Could you check a few things on this model? Use its own coordinates, in mm. Coordinates: 2 decimals unless noted, no trailing zeros. Loops run counter-clockwise (first coordinate to the right, second up) from the corner with the lowest first, then second, coordinate; pieces in that order, holes last. Notation, with made-up numbers: (10, 37.5) - (44, 37.5) arc R21 ccw to (44, 64.5) - close; hole circle Ø6 at (40.25, 61). An arc over 180 degrees is marked (long way). Use CSV: the item, a comma, the result in double quotes.
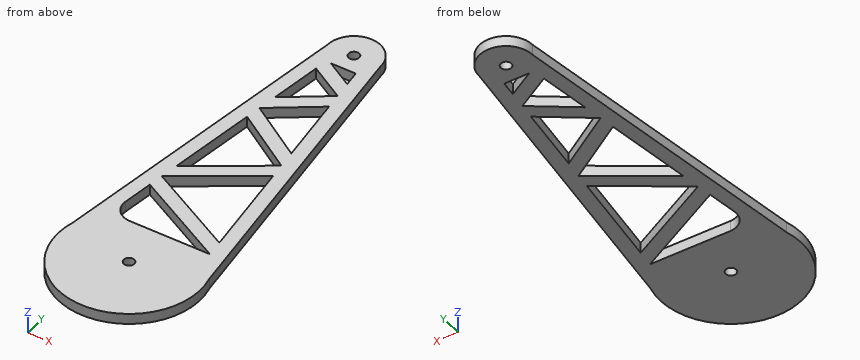
from build123d import *

# Parameters (mm, degrees)
SKETCH1_R           = 1.5
BOSS_EXTRUDE1_DEPTH = 3
FILLET1_R           = 5


with BuildPart() as part:
    # Sketch1 → Boss-Extrude1 (new body)
    with BuildSketch(Plane.XY):
        with BuildLine():
            Line((-19.319264806, 5.173587474), (-7.5, 95))
            ThreePointArc((-7.5, 95), (0, 102.5), (7.5, 95))
            Line((7.5, 95), (19.319264806, 5.173587474))
            ThreePointArc((19.319264806, 5.173587474), (0, -20), (-19.319264806, 5.173587474))
        make_face()
        with Locations((0, 95)):
            Circle(SKETCH1_R, mode=Mode.SUBTRACT)
        Circle(SKETCH1_R, mode=Mode.SUBTRACT)
        Polygon((-14.254996232, 13), (14.254996232, 13), (-12.38556129, 27.207705563), align=None, mode=Mode.SUBTRACT)
        Polygon((-2.898329399, 89.534418399), (4.184678022, 89.534418399), (4.774242146, 85.053731057), align=None, mode=Mode.SUBTRACT)
        Polygon((-11.828187859, 31.443743635), (13.613494732, 17.875411404), (9.904156147, 46.066384645), align=None, mode=Mode.SUBTRACT)
        Polygon((-11.132206149, 36.73320463), (-7.866560771, 61.552109505), (9.321386275, 50.495435676), align=None, mode=Mode.SUBTRACT)
        Polygon((-7.289587852, 65.937103693), (8.637709175, 55.691381633), (6.027006268, 75.532723726), align=None, mode=Mode.SUBTRACT)
        Polygon((-6.572917095, 71.383801447), (5.434465341, 80.036034774), (-4.658887227, 85.930428438), align=None, mode=Mode.SUBTRACT)
    extrude(amount=BOSS_EXTRUDE1_DEPTH)

    # Fillet1
    fillet1_edges = [part.edges().sort_by_distance(p)[0] for p in [
        (-14.254996232, 13, 1.5),
    ]]
    fillet(fillet1_edges, radius=FILLET1_R)


solid = part.part
(1) Suppose I cut it at A-A (y = 0). Write out the boundary of the cut face in (x, z).
Computed:
outline,"(-20, 0) - (-1.5, 0) - (-1.5, 3) - (-20, 3) - close; (1.5, 0) - (20, 0) - (20, 3) - (1.5, 3) - close"
(2) Please list where these lines run through material, in increasing order: line 1 (X direction, y = 95, z = 1.5); line 2 (X direction, y = 40, z = 0.15); line 3 (X direction, y = 45, z = 0.6).
Computed:
line 1,"x = -7.5 to -1.5, 1.5 to 7.5"
line 2,"x = -14.74 to -10.7, -6.28 to 0.89, 10.7 to 14.74"
line 3,"x = -14.08 to -10.04, 1.15 to 8.32, 10.04 to 14.08"
(3) Suppose I cut it at D-D (x = 3). Write out the boundary of the cut face in (y, z).
Computed:
outline,"(-19.77, 0) - (13, 0) - (13, 3) - (-19.77, 3) - close; (19, 0) - (23.54, 0) - (23.54, 3) - (19, 3) - close; (41.42, 0) - (46.24, 0) - (46.24, 3) - (41.42, 3) - close; (54.56, 0) - (59.32, 0) - (59.32, 3) - (54.56, 3) - close; (73.35, 0) - (78.28, 0) - (78.28, 3) - (73.35, 3) - close; (81.46, 0) - (86.09, 0) - (86.09, 3) - (81.46, 3) - close; (89.53, 0) - (101.87, 0) - (101.87, 3) - (89.53, 3) - close"
(4) Will these pins go through, and if not, where does the flat tip stop? pin 1 (1.5 mm diameter, centred on y = 56, z = 1, fed in from +X); pin 2 (1.5 mm diameter, centred on y = 78, z = 1.5, fed in from +X); pin 3 (0.9 mm diameter, centred on x = 6, z = 1, fed in from +Y).
Computed:
pin 1,"stops at x = 12.73"
pin 2,"stops at x = 9.84"
pin 3,"stops at y = 100.04"
(5) Suppose I cut it at B-B (x = -10). Write out the boundary of the cut face in (y, z), plus the area to 3 significant figures.
Computed:
outline,"(-17.32, 0) - (13.21, 0) - (13.21, 3) - (-17.32, 3) - close; (25.94, 0) - (30.47, 0) - (30.47, 3) - (25.94, 3) - close; (32.67, 0) - (37.5, 0) - (37.5, 3) - (32.67, 3) - close; (45.34, 0) - (76, 0) - (76, 3) - (45.34, 3) - close"
area,"212 mm²"
(6) Suppose I cut it at C-C (z = 1.15). State how many separate pieces and enclosed holes the cut face has, plus the area to 3 significant figures.
Computed:
separate pieces,"1"
enclosed holes,"8"
area,"2,320 mm²"
